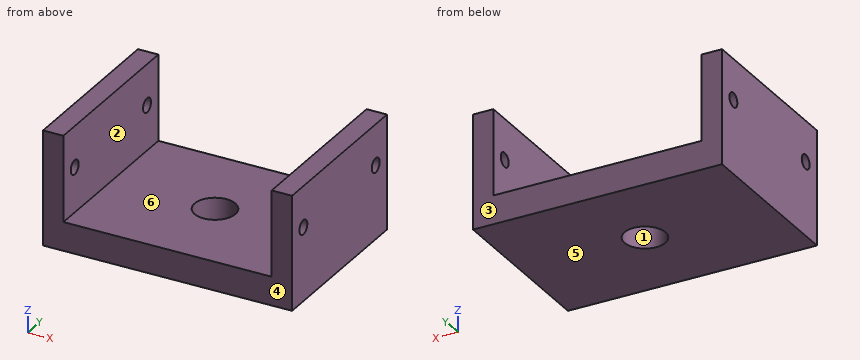
```python
from build123d import *

# Parameters (mm, degrees)
SKETCH1_W           = 61
SKETCH1_H           = 42
SKETCH1_R           = 5
BOSS_EXTRUDE1_DEPTH = 7
SKETCH2_W           = 5
SKETCH2_H           = 42
BOSS_EXTRUDE2_DEPTH = 21
SKETCH3_R           = 1.75
CUT_EXTRUDE1_DEPTH  = 71.32780389


with BuildPart() as part:
    # Sketch1 → Boss-Extrude1 (new body)
    with BuildSketch(Plane.XY):
        Rectangle(SKETCH1_W, SKETCH1_H)
        Circle(SKETCH1_R, mode=Mode.SUBTRACT)
    extrude(amount=BOSS_EXTRUDE1_DEPTH)

    # Sketch2 → Boss-Extrude2 (add)
    with BuildSketch(Plane.XY.offset(7)):
        with Locations((-28, 0)):
            Rectangle(SKETCH2_W, SKETCH2_H)
        with Locations((28, 0)):
            Rectangle(SKETCH2_W, SKETCH2_H)
    extrude(amount=BOSS_EXTRUDE2_DEPTH)

    # Sketch3 → Cut-Extrude1 (cut, through all)
    with BuildSketch(Plane(origin=(30.5, 0, 0), x_dir=(0, 0, -1), z_dir=(1, 0, 0))):
        with Locations(Location((-18, 16, 0), (0, 0, 90))):
            Circle(SKETCH3_R)
        with Locations((-18, -16)):
            Circle(SKETCH3_R)
    extrude(amount=-CUT_EXTRUDE1_DEPTH, mode=Mode.SUBTRACT)


solid = part.part
```
Work out the finished part from the listing and answer in its coordinate system (mm). Face numbers are marked on the shaded views. A direction names the side the tool comes from. Round coordinates to 2 decimals unless told otherwise and drop trailing zeros. Order: outer loops, then holes, each group sorted by start corner. A loop starts at its lowest first (then second) coordinate and runs counter-clockwise, first axis right, second up.
Q1. A cutting plane is placed at A-A, the plane y = 16. Determine the outline of the cut face in (x, z), then the cut area to 3 significant figures.
Solution:
outline: (-30.5, 0) - (30.5, 0) - (30.5, 16.25) - (25.5, 16.25) - (25.5, 7) - (-25.5, 7) - (-25.5, 16.25) - (-30.5, 16.25) - close; (-30.5, 19.75) - (-25.5, 19.75) - (-25.5, 28) - (-30.5, 28) - close; (25.5, 19.75) - (30.5, 19.75) - (30.5, 28) - (25.5, 28) - close
area: 602 mm2
Q2. Find the intervals of material crossed by line 1 along X through (y, z) = (3, 14.5); line 2 along Z through (x, y) = (27.4, 16); line 3 along Y through (x, z) = (-2, 5.5), in increasing order.
Solution:
line 1: x = -30.5 to -25.5, 25.5 to 30.5
line 2: z = 0 to 16.25, 19.75 to 28
line 3: y = -21 to -4.58, 4.58 to 21
Q3. A tool of negligible diameter and unlimited length cuts with its end or side. For the marked faces 5 and 6, from which of +Z, -Z, +X, -X, +Y, -Y can it reach the whole face along a straight path? Write none if from no direction.
Solution:
face 5: -Z, +X, -X, +Y, -Y
face 6: +Z, +Y, -Y
Q4. A cutting plane is placed at C-C, the plane y = 0. Determine the outline of the cut face in (x, z).
Solution:
outline: (-30.5, 0) - (-5, 0) - (-5, 7) - (-25.5, 7) - (-25.5, 28) - (-30.5, 28) - close; (5, 0) - (30.5, 0) - (30.5, 28) - (25.5, 28) - (25.5, 7) - (5, 7) - close
Q5. A cutting plane is placed at B-B, the plane z = 10. Determine the outline of the cut face in (x, y), then the cut area to 3 significant figures.
Solution:
outline: (-30.5, -21) - (-25.5, -21) - (-25.5, 21) - (-30.5, 21) - close; (25.5, -21) - (30.5, -21) - (30.5, 21) - (25.5, 21) - close
area: 420 mm2
Q6. The mould has two halves that part along Y. Classify the marked faces 1, 2, 3 and 4: pulls with the +Y half, pulls with the -Y half, needs draft (parallel to the pull), parting line crosses it, or undercut.
Solution:
face 1: undercut
face 2: needs draft
face 3: pulls with the +Y half
face 4: pulls with the -Y half
Q7. A cutting plane is placed at D-D, the plane x = 0. Determine the outline of the cut face in (y, z), then the cut area to 3 significant figures.
Solution:
outline: (-21, 0) - (-5, 0) - (-5, 7) - (-21, 7) - close; (5, 0) - (21, 0) - (21, 7) - (5, 7) - close
area: 224 mm2
Q8. Given pin 1 Ø5.5 at (y, z) = (16, 18) entering from -X; pin 2 Ø6 at (x, y) = (10.5, 7.5) entering from +Z, each flat-ended and moving along its own axis, determine where each tip first touches the part or whether it passes through.
Solution:
pin 1: stops at x = -30.5
pin 2: stops at z = 7
